Geometry: final body of the model. Coordinates: model frame, mm. Round coordinates to 2 decimals unless told otherwise and drop trailing zeros. Loops run counter-clockwise (first coordinate to the right, second up) from the corner with the lowest first, then second, coordinate; pieces in that order, holes last. Notation, with made-up numbers: (15, 69.5) -> (57, 69.5) arc R14 cw to (57, 79.5) -> close; hole circle Ø7 at (48.5, 16). An arc over 180 degrees is marked (long way). Answer in a Markdown table with one row per item.
```python
from build123d import *

# Parameters (mm, degrees)
F1_DEPTH = 6.35


with BuildPart() as f1:
    # F0 (on Top) → F1 (new body)
    with BuildSketch(Plane.XY):
        with BuildLine():
            Line((76.2, 0), (12.7, 0))
            ThreePointArc((12.7, 0), (3.719744, -3.719744), (0, -12.7))
            Line((0, -12.7), (0, -139.7))
            ThreePointArc((0, -139.7), (3.719744, -148.680256), (12.7, -152.4))
            Line((12.7, -152.4), (76.2, -152.4))
            Line((76.2, -152.4), (76.2, -101.981))
            ThreePointArc((76.2, -101.981), (50.419, -76.2), (76.2, -50.419))
            Line((76.2, -50.419), (76.2, 0))
        make_face()
        with BuildLine():
            Line((139.7, 0), (76.2, 0))
            Line((76.2, 0), (76.2, -50.419))
            ThreePointArc((76.2, -50.419), (94.42992, -57.97008), (101.981, -76.2))
            ThreePointArc((101.981, -76.2), (94.42992, -94.42992), (76.2, -101.981))
            Line((76.2, -101.981), (76.2, -152.4))
            Line((76.2, -152.4), (139.7, -152.4))
            ThreePointArc((139.7, -152.4), (148.680256, -148.680256), (152.4, -139.7))
            Line((152.4, -139.7), (152.4, -12.7))
            ThreePointArc((152.4, -12.7), (148.680256, -3.719744), (139.7, 0))
        make_face()
    extrude(amount=F1_DEPTH)


solid = f1.part
```
Item 1: Cut plane C-C (x = 78). Output: boundary loops of the cut face in (y, z), then the cut area to 3 significant figures.
Answer:
| item | result |
|---|---|
| outline | (-152.4, 0) -> (-101.92, 0) -> (-101.92, 6.35) -> (-152.4, 6.35) -> close; (-50.48, 0) -> (0, 0) -> (0, 6.35) -> (-50.48, 6.35) -> close |
| area | 641 mm² |
Item 2: Cut plane B-B (y = -72.5). Output: boundary loops of the cut face in (x, z).
Answer:
| item | result |
|---|---|
| outline | (0, 0) -> (50.69, 0) -> (50.69, 6.35) -> (0, 6.35) -> close; (101.71, 0) -> (152.4, 0) -> (152.4, 6.35) -> (101.71, 6.35) -> close |
Item 3: Cut plane A-A (z = 1.5). Output: boundary loops of the cut face in (x, y).
Answer:
| item | result |
|---|---|
| outline | (0, -139.7) arc R12.7 ccw to (12.7, -152.4) -> (139.7, -152.4) arc R12.7 ccw to (152.4, -139.7) -> (152.4, -12.7) arc R12.7 ccw to (139.7, 0) -> (12.7, 0) arc R12.7 ccw to (0, -12.7) -> close; hole circle Ø51.56 at (76.2, -76.2) |
Item 4: Line query: probe 1 along Y at (x, z) = (140.5, 3.25); probe 2 along Y at (x, z) = (88, 2); probe 3 along Y at (x, z) = (84.5, 2). Output: solid intervals per line, ascending. Write a range as [from, to].
Answer:
| item | result |
|---|---|
| probe 1 | y = [-152.37, -0.03] |
| probe 2 | y = [-152.4, -99.12], [-53.28, 0] |
| probe 3 | y = [-152.4, -100.61], [-51.79, 0] |
